from build123d import *

# Parameters (mm, degrees)
SKETCH1_W            = 36
SKETCH1_H            = 110
BOSS_EXTRUDE1_DEPTH  = 1
M3_CLEARANCE_HOLE1_D = 3.4
M4_CLEARANCE_HOLE1_D = 4.5
M3_CLEARANCE_HOLE2_D = 3.4
BOSS_EXTRUDE2_DEPTH  = 1


with BuildPart() as part:
    # Sketch1 → Boss-Extrude1 (new body)
    with BuildSketch(Plane(origin=(0, 0, 0), x_dir=(0, 0, -1), z_dir=(1, 0, 0))):
        with Locations((0, -55)):
            Rectangle(SKETCH1_W, SKETCH1_H)
    extrude(amount=BOSS_EXTRUDE1_DEPTH)

    # M3 Clearance Hole1 (through all)
    with Locations(Plane.ZY):
        with Locations((-10, -10), (10, -10)):
            Hole(M3_CLEARANCE_HOLE1_D / 2)

    # M4 Clearance Hole1 (through all)
    with Locations(Plane.ZY):
        with Locations((-13, -19), (13, -19)):
            Hole(M4_CLEARANCE_HOLE1_D / 2)

    # M3 Clearance Hole2 (through all)
    with Locations(Plane(origin=(1, 0, 0), x_dir=(0, 0, -1), z_dir=(1, 0, 0))):
        with Locations((6, -104), (-6, -104), (6, -94), (-6, -94), (6, -84), (-6, -84), (6, -74), (-6, -74), (6, -64), (-6, -64), (6, -54), (-6, -54), (6, -44), (-6, -44), (6, -34), (-6, -34)):
            Hole(M3_CLEARANCE_HOLE2_D / 2)

    # Sketch9 → Boss-Extrude2 (add)
    with BuildSketch(Plane.ZY):
        with BuildLine():
            Line((18, -25.35), (22.885533906, -30.235533906))
            ThreePointArc((22.885533906, -30.235533906), (23.969397663, -31.85765065), (24.35, -33.771067812))
            Line((24.35, -33.771067812), (24.35, -105))
            ThreePointArc((24.35, -105), (22.885533906, -108.535533906), (19.35, -110))
            Line((19.35, -110), (18, -110))
            Line((18, -110), (18, -25.35))
        make_face()
        with BuildLine():
            Line((-18, -25.35), (-22.885533906, -30.235533906))
            ThreePointArc((-22.885533906, -30.235533906), (-23.969397663, -31.85765065), (-24.35, -33.771067812))
            Line((-24.35, -33.771067812), (-24.35, -105))
            ThreePointArc((-24.35, -105), (-22.885533906, -108.535533906), (-19.35, -110))
            Line((-19.35, -110), (-18, -110))
            Line((-18, -110), (-18, -25.35))
        make_face()
    extrude(amount=-BOSS_EXTRUDE2_DEPTH)


solid = part.part
Geometry check sheet. Reference: the model listing, model coordinates, mm. Coordinates: 2 decimals unless noted, no trailing zeros. Order: outer loops, then holes, each group sorted by start corner. A loop starts at its lowest first (then second) coordinate and runs counter-clockwise, first axis right, second up. Notation, with made-up numbers: (9, 41) - (26, 41) arc R21 cw to (26, 74) - close; hole circle Ø9 at (47.5, -11). An arc over 180 degrees is marked (long way). One line per item, written item: value.
(1) Sectioned sample at C-C (y = -19). Enter the section's corners in (x, z), and give its area (3 significant figures).
Data:
outline: (0, -18) - (1, -18) - (1, -15.25) - (0, -15.25) - close; (0, -10.75) - (1, -10.75) - (1, 10.75) - (0, 10.75) - close; (0, 15.25) - (1, 15.25) - (1, 18) - (0, 18) - close
area: 27.0 mm^2
(2) Sectioned sample at A-A (y = -54). Enter the section's corners in (x, z).
Data:
outline: (0, -24.35) - (1, -24.35) - (1, -7.7) - (0, -7.7) - close; (0, -4.3) - (1, -4.3) - (1, 4.3) - (0, 4.3) - close; (0, 7.7) - (1, 7.7) - (1, 24.35) - (0, 24.35) - close
(3) Sectioned sample at B-B (z = -13). Enter the section's corners in (x, y).
Data:
outline: (0, -110) - (1, -110) - (1, -21.25) - (0, -21.25) - close; (0, -16.75) - (1, -16.75) - (1, 0) - (0, 0) - close
(4) Depth check by flat-ended pin: pin 1 Ø2.5 at (y, z) = (-94, -6) entering from -X; pin 2 Ø0.5 at (x, y) = (0.5, -14.5) entering from +Z. Enter the tip coordinate at first touch or a pass-through.
Data:
pin 1: passes through
pin 2: stops at z = 18
(5) Sectioned sample at D-D (z = -6). Count the separate pieces of the cut face and the enclosed holes in it, and give its area (3 significant figures).
Data:
separate pieces: 9
enclosed holes: 0
area: 82.8 mm^2
(6) Thickness scan on probe 1 along Z at (x, y) = (0.45, -84); probe 2 along Y at (x, z) = (0.3, -10); probe 3 along Z at (x, y) = (0.15, -103.5). Record the ranges inside material, lowest first. Write a range as from..to.
Data:
probe 1: z = -24.35..-7.7, -4.3..4.3, 7.7..24.35
probe 2: y = -110..-11.7, -8.3..0
probe 3: z = -24.35..-7.62, -4.38..4.38, 7.62..24.35
